The model under review builds one solid part; all positions refer to its coordinate system, in mm. Face numbers are marked on the shaded views. A direction names the side the tool comes from. Round coordinates to 2 decimals unless told otherwise and drop trailing zeros. Write each loop counter-clockwise with the first axis right and the second up, starting at its lowest first coordinate (ties: lowest second). Pieces come first, ordered by that corner, then holes. Notation, with made-up numbers: (1.5, 87.25) -> (40.5, 87.25) arc R14 ccw to (40.5, 105.25) -> close; hole circle Ø11 at (43, 40). An arc over 180 degrees is marked (long way). Use CSV: the item, a comma, the result in double quotes. Start each with the question number.
1) Take a section at C-C, the plane x = -12. Give the boundary of the cut face in (y, z).
2) For pin 1 Ø1.5 at (x, y) = (-34.5, 26) entering from -Z; pin 2 Ø4 at (x, y) = (-37, 26) entering from +Z; pin 3 Ø6 at (x, z) = (-27, -8) entering from +Y, all flat-tipped, find the tip position at first contact; note any pin that passes through.
3) Take a section at B-B, the plane y = 19.5. Give the boundary of the cut face in (x, z).
4) Take a section at D-D, the plane z = -24.25. Give the boundary of the cut face in (x, y), then the cut area to 3 significant figures.
5) Wall thickness on probe 1 along Z at (x, y) = (-6, 16); probe 2 along X at (y, z) = (18.75, -22); probe 3 along X at (y, z) = (24.5, -18.25): over which ranges is each line inside the solid? List them lowest first. Write a range as [from, to].
6) Mouldability with a two-part tool opening along X and no side actions: class the marked faces 5, 6 and 7 as released by +X, released by -X, zero draft, split by the parting line, or undercut.
7) Machinability: for the marked faces 1, 2, 3 and 4, which of the approach directions +Z, -Z, +X, -X, +Y, -Y give a long, thin tool a straight path to every point of the face, cutting with its end or side? Answer none if there is none.
8) Take a section at A-A, the plane z = -10.5. Give the boundary of the cut face in (x, y).
Autodesk Inventor part; units mm, degrees
ref_plane "YZ Plane" through (0, 0, 0) normal (1, 0, 0) x (0, 1, 0)
ref_plane "XZ Plane" through (0, 0, 0) normal (0, 1, 0) x (-1, 0, 0)
ref_plane "XY Plane" through (0, 0, 0) normal (0, 0, 1) x (1, 0, 0)
sketch "Эскиз1" plane through (0, 0, 0) normal (0, 1, 0) x (-1, 0, 0)
  line L0 (0, 0) -> (47, 0)
  line L1 (47, 0) -> (47, -27)
  line L2 (47, -27) -> (0, -27)
  line L3 (0, -27) -> (0, 0)
  dimension "d0" = 47
  dimension "d1" = 27
extrude "Выдавливание1" add sketch "Эскиз1" along normal blind 22.5
sketch "Эскиз2" plane through (0, 22.5, 0) normal (0, 1, 0) x (1, 0, 0)
  line L0 (-18, 1.5) -> (-1.5, 1.5)
  line L1 (-1.5, 1.5) -> (-1.5, 25.5)
  line L2 (-1.5, 25.5) -> (-18, 25.5)
  line L3 (-18, 25.5) -> (-18, 1.5)
  line L4 (-47, 0) -> (0, 0)
  line L5 (0, 0) -> (0, 27)
  dimension "d4" = 16.5
  dimension "d5" = 24
  dimension "d6" = 1.5
  dimension "d7" = 1.5
extrude "Выдавливание2" cut sketch "Эскиз2" against normal blind 15.5
sketch "Эскиз3" plane through (0, 22.5, 0) normal (0, 1, 0) x (1, 0, 0)
  line L0 (-41, 6) -> (-31, 6)
  line L1 (-31, 6) -> (-31, 21)
  line L2 (-31, 21) -> (-41, 21)
  line L3 (-41, 21) -> (-41, 6)
  line L4 (-47, 27) -> (-47, 0)
  line L5 (-47, 0) -> (0, 0)
  dimension "d10" = 10
  dimension "d11" = 15
  dimension "d12" = 6
  dimension "d13" = 6
extrude "Выдавливание3" add sketch "Эскиз3" along normal blind 5
properties part number "Разъем220"
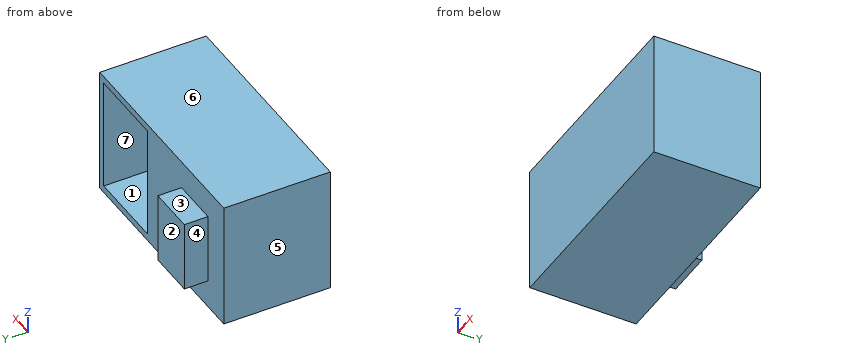
Values found:
1,outline,"(0, -27) -> (22.5, -27) -> (22.5, -25.5) -> (7, -25.5) -> (7, -1.5) -> (22.5, -1.5) -> (22.5, 0) -> (0, 0) -> close"
2,pin 1,"z = -21"
2,pin 2,"z = -6"
2,pin 3,"y = 22.5"
3,outline,"(-47, -27) -> (0, -27) -> (0, 0) -> (-47, 0) -> close; hole (-18, -25.5) -> (-1.5, -25.5) -> (-1.5, -1.5) -> (-18, -1.5) -> close"
4,outline,"(-47, 0) -> (0, 0) -> (0, 22.5) -> (-1.5, 22.5) -> (-1.5, 7) -> (-18, 7) -> (-18, 22.5) -> (-47, 22.5) -> close"
4,area,"802 mm²"
5,probe 1,"[-27, -25.5], [-1.5, 0]"
5,probe 2,"[-47, -18], [-1.5, 0]"
5,probe 3,"[-41, -31]"
6,face 5,"released by -X"
6,face 6,"zero draft"
6,face 7,"undercut"
7,face 1,"+Y"
7,face 2,"+Z, -Z, +X, -X, +Y"
7,face 3,"+Z, +X, -X, +Y"
7,face 4,"+Z, -Z, -X, +Y"
8,outline,"(-47, 0) -> (0, 0) -> (0, 22.5) -> (-1.5, 22.5) -> (-1.5, 7) -> (-18, 7) -> (-18, 22.5) -> (-31, 22.5) -> (-31, 27.5) -> (-41, 27.5) -> (-41, 22.5) -> (-47, 22.5) -> close"
